from build123d import *

# Parameters (mm, degrees)
SALIENTE_EXTRUIR1_DEPTH = 50.8
CROQUIS6_R              = 6.35
CORTAR_EXTRUIR1_DEPTH   = 10


with BuildPart() as part:
    # Croquis1 → Saliente-Extruir1 (new body)
    with BuildSketch(Plane(origin=(0, 0, 0), x_dir=(0, 0, -1), z_dir=(1, 0, 0))):
        Polygon((-6.31, 93.46), (0, 93.46), (0, 0), (-962, 0), (-962, 6.31), (-6.31, 6.31), align=None)
    extrude(amount=SALIENTE_EXTRUIR1_DEPTH)

    # Croquis6 → Cortar-Extruir1 (cut)
    with BuildSketch(Plane.XZ):
        with Locations(Location((25.4, 918.107795334, 0), (0, 0, 270))):
            Circle(CROQUIS6_R)
        with Locations(Location((25.4, 950.107795334, 0), (0, 0, 270))):
            Circle(CROQUIS6_R)
    extrude(amount=-CORTAR_EXTRUIR1_DEPTH, mode=Mode.SUBTRACT)


solid = part.part
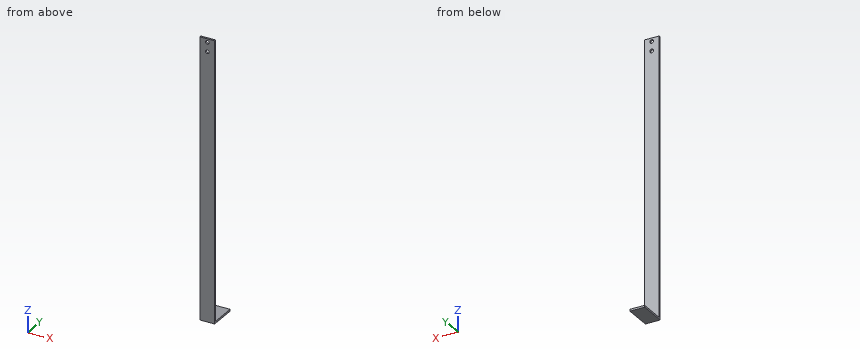
The model under review builds one solid part; all positions refer to its coordinate system, in mm. Round coordinates to 2 decimals unless told otherwise and drop trailing zeros. Loops run counter-clockwise (first coordinate to the right, second up) from the corner with the lowest first, then second, coordinate; pieces in that order, holes last. Notation, with made-up numbers: M -15,10 L 3,10 A4 cw 3,15 Z; hole C 6,5 d11. An arc over 180 degrees is marked long. Answer as a JSON object with one key per item and string values.
Item 1: We need section A-A, the plane y = 74. State the section outline as (x, z) points.
Check sheet entries:
{"outline": "M 0,0 L 50.8,0 L 50.8,6.31 L 0,6.31 Z"}
Item 2: For line 1 along Z through (x, y) = (25, 2); line 2 along Y through (x, z) = (3, 185), list the stretches that pass through material, from the lowest coordinate up.
Check sheet entries:
{"line 1": "0 to 911.77, 924.45 to 943.77, 956.45 to 962", "line 2": "0 to 6.31"}
Item 3: Clearance check with flat-ended pins moving along their axes: P1, Ø1, axis at x = 37.5, z = 110.5, coming from the -Y side; P2, Ø5, axis at x = 28.5, z = 224.5, coming from the +Y side; P3, Ø6, axis at x = 25, y = 52, coming from the +Z side. State where each tip first meets the part, or that it passes through.
Check sheet entries:
{"P1": "y = 0", "P2": "y = 6.31", "P3": "z = 6.31"}
